```python
from build123d import *

# Parameters (mm, degrees)
BOSS_EXTRUDE1_DEPTH = 3.96875
SKETCH2_W           = 89.725
SKETCH2_H           = 14.7
BOSS_EXTRUDE2_DEPTH = 2
SKETCH3_R           = 3.25
CUT_EXTRUDE1_DEPTH  = 92.116911721
SKETCH4_W           = 2
SKETCH4_H           = 14.7
SKETCH4_W_2         = 30
SKETCH4_H_2         = 2
BOSS_EXTRUDE3_DEPTH = 2.4


with BuildPart() as part:
    # Sketch1 → Boss-Extrude1 (new body)
    with BuildSketch(Plane(origin=(0, 0, 0), x_dir=(1, 0, 0), z_dir=(0, 1, 0))):
        Polygon((0, 0), (0, 14.7), (89.725, 14.7), (89.725, 0), (87.725, 0), (87.725, 12.7), (2, 12.7), (2, 0), align=None)
    extrude(amount=BOSS_EXTRUDE1_DEPTH)

    # Sketch2 → Boss-Extrude2 (add)
    with BuildSketch(Plane(origin=(0, 3.96875, 0), x_dir=(1, 0, 0), z_dir=(0, 1, 0))):
        with Locations((44.8625, 7.35)):
            Rectangle(SKETCH2_W, SKETCH2_H)
    extrude(amount=BOSS_EXTRUDE2_DEPTH)

    # Sketch3 → Cut-Extrude1 (cut, through all)
    with BuildSketch(Plane(origin=(0, 5.96875, 0), x_dir=(1, 0, 0), z_dir=(0, 1, 0))):
        with Locations(Location((17.95, 5.25, 0), (0, 0, 270))):
            Circle(SKETCH3_R)
        with Locations(Location((26.45, 5.25, 0), (0, 0, 270))):
            Circle(SKETCH3_R)
        with Locations(Location((34.95, 5.25, 0), (0, 0, 270))):
            Circle(SKETCH3_R)
        with Locations(Location((43.45, 5.25, 0), (0, 0, 270))):
            Circle(SKETCH3_R)
        with Locations(Location((51.95, 5.25, 0), (0, 0, 270))):
            Circle(SKETCH3_R)
    extrude(amount=-CUT_EXTRUDE1_DEPTH, mode=Mode.SUBTRACT)

    # Sketch4 → Boss-Extrude3 (add)
    with BuildSketch(Plane(origin=(0, 0, 0), x_dir=(-1, 0, 0), z_dir=(0, -1, 0))):
        with Locations((-88.725, 7.35)):
            Rectangle(SKETCH4_W, SKETCH4_H)
        with Locations((-1, 7.35)):
            Rectangle(SKETCH4_W, SKETCH4_H)
        with Locations((-44.8625, 13.7)):
            Rectangle(SKETCH4_W_2, SKETCH4_H_2)
    extrude(amount=BOSS_EXTRUDE3_DEPTH)


solid = part.part
```
CAD build for the part. Positions are in the model's coordinates, mm. A direction names the side the tool comes from. Coordinates: 2 decimals unless noted, no trailing zeros. Order: outer loops, then holes, each group sorted by start corner. A loop starts at its lowest first (then second) coordinate and runs counter-clockwise, first axis right, second up. Notation, with made-up numbers: M 13,81 L 60,81 A26 cw 60,102 Z; hole C 23.5,29.5 d4. An arc over 180 degrees is marked long. Answer as CSV lines item,"result".
1) Cut at B-B (y = -1). List the corners of the cut face in (x, z) (1 decimal).
Verdict:
outline,"M 0,-14.7 L 2,-14.7 L 2,0 L 0,0 Z; M 29.9,-14.7 L 59.9,-14.7 L 59.9,-12.7 L 29.9,-12.7 Z; M 87.7,-14.7 L 89.7,-14.7 L 89.7,0 L 87.7,0 Z"
2) Cut at A-A (x = 34.95). List the corners of the cut face in (y, z).
Verdict:
outline,"M -2.4,-14.7 L 5.97,-14.7 L 5.97,-8.5 L 3.97,-8.5 L 3.97,-12.7 L -2.4,-12.7 Z; M 3.97,-2 L 5.97,-2 L 5.97,0 L 3.97,0 Z"
3) Cut at C-C (z = -5.25). List the corners of the cut face in (x, y) (3 decimals).
Verdict:
outline,"M 0,-2.4 L 2,-2.4 L 2,3.969 L 14.7,3.969 L 14.7,5.969 L 0,5.969 Z; M 21.2,3.969 L 23.2,3.969 L 23.2,5.969 L 21.2,5.969 Z; M 29.7,3.969 L 31.7,3.969 L 31.7,5.969 L 29.7,5.969 Z; M 38.2,3.969 L 40.2,3.969 L 40.2,5.969 L 38.2,5.969 Z; M 46.7,3.969 L 48.7,3.969 L 48.7,5.969 L 46.7,5.969 Z; M 55.2,3.969 L 87.725,3.969 L 87.725,-2.4 L 89.725,-2.4 L 89.725,5.969 L 55.2,5.969 Z"
4) Flat gauge pins, fed straight in: P1, Ø5, axis at x = 43.45, z = -5.25, coming from the -Y side; P2, Ø2, axis at x = 72.5, z = -11.5, coming from the -Y side; P3, Ø1, axis at x = 76.5, z = -13.5, coming from the -Y side. Where does each tip first touch, or does it go through?
Verdict:
P1,"through"
P2,"y = 3.97"
P3,"y = 0"
5) Mould opens along X. For faces 1 (the flat face through (0, 2, -7)), 2 (the flat face through (74, 0, -14)), 3 (the flat face through (89.725, 2, -7)) say: released by +X, released by -X, zero draft, split by the parting line, or undercut.
Verdict:
face 1,"released by -X"
face 2,"undercut"
face 3,"released by +X"
6) 3-axis set-ups, long thin cutter, end or side, ignore diameter. For faces 4 (the flat face through (1, -2.4, -7)), 5 (the flat face through (29.862, -1, -14)), 6 (the flat face through (87.725, 1, -7)): which of +Z, -Z, +X, -X, +Y, -Y reach the whole face in a straight line?
Verdict:
face 4,"+Z, -Z, +X, -X, -Y"
face 5,"+Z, -Z, -Y"
face 6,"+Z, -Y"
7) Drill centre lines: L1, parallel to X at y = 4.7, z = -5.25 (3 decimals); L2, parallel to X at y = 1.5, z = -11.5 (3 decimals); L3, parallel to Z at x = 26.5, y = 5.5. Where is each one in solid material? Low to high. Write a range as from..to.
Verdict:
L1,"0..14.7, 21.2..23.2, 29.7..31.7, 38.2..40.2, 46.7..48.7, 55.2..89.725"
L2,"0..2, 87.725..89.725"
L3,"-14.7..-8.5, -2..0"
8) Cut at D-D (y = 2.25). List the corners of the cut face in (x, z) (3 decimals), then the cut area to 3 significant figures.
Verdict:
outline,"M 0,-14.7 L 89.725,-14.7 L 89.725,0 L 87.725,0 L 87.725,-12.7 L 2,-12.7 L 2,0 L 0,0 Z"
area,"230 mm2"
